Source: three-view drawing plus pictorial views. Frame: mm from the lowest corner of the part. A direction names the side the tool comes from. Coordinates: 2 decimals unless noted, no trailing zeros. Loops run counter-clockwise (first coordinate to the right, second up) from the corner with the lowest first, then second, coordinate; pieces in that order, holes last.
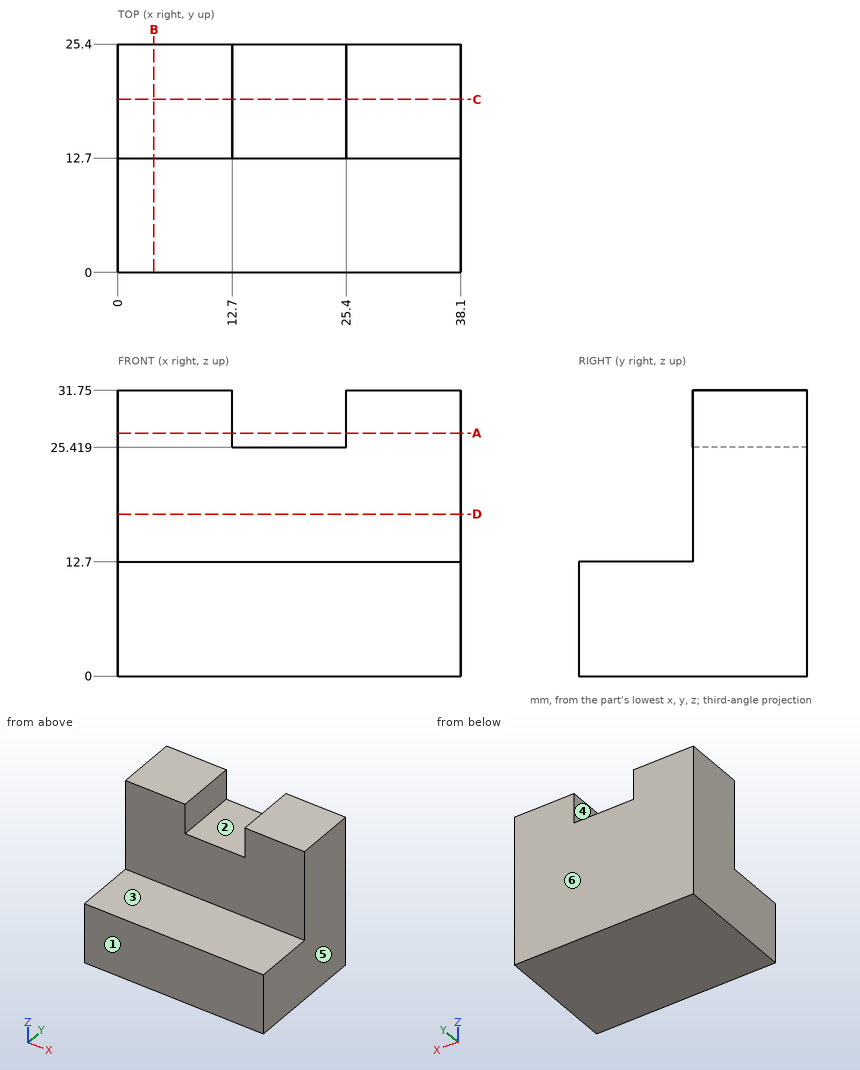
Q1. Section D-D, the plane z = 18. Return the cut outline in (x, y).
Q2. Section C-C, the plane y = 19.25. Return the cut outline in (x, z).
Q3. Section A-A, the plane z = 27. Return the cut outline in (x, y), plus the area to 3 significant figures.
Q4. Section B-B, the plane x = 4. Return the cut outline in (y, z), plus the area to 4 significant figures.
Q5. Draft query along X for the marked faces 4, 5 and 6. Return one class per face: +X half, -X half, draft (parallel to the pull), parting line (faces both ways), or undercut.
Q6. Contact query for flat-ended pins moving along their axis: pin 1 Ø2 at (x, y) = (17.5, 11) entering from +Z; pin 2 Ø4 at (x, z) = (24.5, 22) entering from -Y. Output: stop coordinate, or through.
Q7. Access query for the marked faces 1, 2 and 3. Directions: +Z, -Z, +X, -X, +Y, -Y. A direction counts if a zero-diameter tool reaches every point of the face in a straight line with its end or side. Return the directions, or none.
Q8. Line query: line 1 along X through (y, z) = (23.75, 28); line 2 along Z through (x, y) = (20, 7); line 3 along Y through (x, z) = (19.5, 14). Output: solid intervals per line, ascending.
Derived:
1. outline: (0, 12.7) - (38.1, 12.7) - (38.1, 25.4) - (0, 25.4) - close
2. outline: (0, 0) - (38.1, 0) - (38.1, 31.75) - (25.4, 31.75) - (25.4, 25.42) - (12.7, 25.42) - (12.7, 31.75) - (0, 31.75) - close
3. outline: (0, 12.7) - (12.7, 12.7) - (12.7, 25.4) - (0, 25.4) - close; (25.4, 12.7) - (38.1, 12.7) - (38.1, 25.4) - (25.4, 25.4) - close
3. area: 323 mm2
4. outline: (0, 0) - (25.4, 0) - (25.4, 31.75) - (12.7, 31.75) - (12.7, 12.7) - (0, 12.7) - close
4. area: 564.5 mm2
5. face 4: undercut
5. face 5: +X half
5. face 6: draft
6. pin 1: stops at z = 12.7
6. pin 2: stops at y = 12.7
7. face 1: +Z, -Z, +X, -X, -Y
7. face 2: +Z, +Y, -Y
7. face 3: +Z, +X, -X, -Y
8. line 1: x = 0 to 12.7, 25.4 to 38.1
8. line 2: z = 0 to 12.7
8. line 3: y = 12.7 to 25.4
